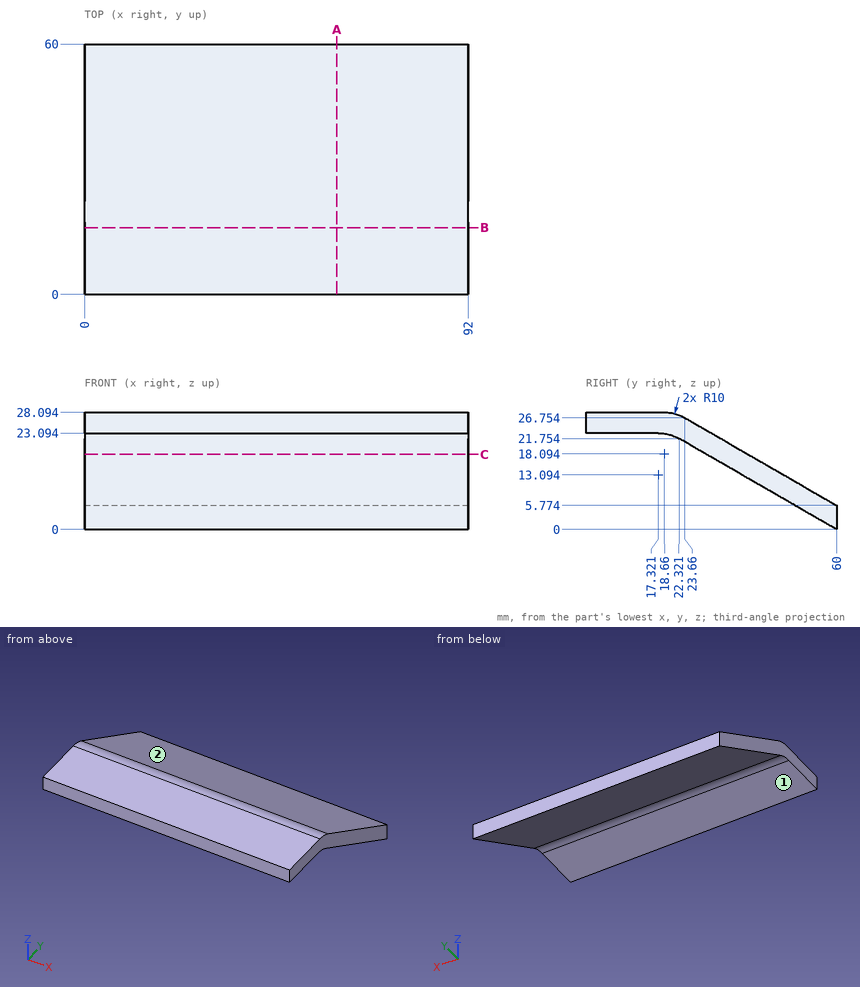
Part print with two shaded views. Sizes in mm from the minimum x, y, z corner. A direction names the side the tool comes from. Give positions to 0.01 mm unless a question says otherwise; leave off trailing zeros. Order: outer loops, then holes, each group sorted by start corner. A loop starts at its lowest first (then second) coordinate and runs counter-clockwise, first axis right, second up.
1) Pin check, flat tips, straight feed: pin 1 (6 mm diameter, centred on x = 39.5, y = 9.5, fed in from -Z); pin 2 (1.5 mm diameter, centred on x = 15, z = 14, fed in from +Y); pin 3 (4 mm diameter, centred on x = 48.5, z = 18, fed in from +Y) (1 decimal). Stop position of each tip, or through.
2) Saw through at A-A, the plane x = 60.5. Write the cut outline in (y, z) (1 decimal).
3) Wall check: probe 1 along Z at (x, y) = (60, 16.5) (1 decimal); probe 2 along Y at (x, z) = (33, 18.25); probe 3 along Z at (x, y) = (69.5, 22.5). Give the ranges that are in metal, low to high.
4) 3-axis set-ups, long thin cutter, end or side, ignore diameter. For the marked faces 1 and 2: which of +Z, -Z, +X, -X, +Y, -Y reach the whole face in a straight line?
5) Saw through at B-B, the plane y = 16. Write the cut outline in (x, z) (1 decimal).
6) Saw through at C-C, the plane z = 18. Write the cut outline in (x, y).
Computed:
1. pin 1: stops at z = 23.09
1. pin 2: stops at y = 47.05
1. pin 3: stops at y = 42.3
2. outline: (0, 23.1) - (17.3, 23.1) arc R10 cw to (22.3, 21.8) - (60, 0) - (60, 5.8) - (23.7, 26.8) arc R10 ccw to (18.7, 28.1) - (0, 28.1) - close
3. probe 1: z = 23.1 to 28.1
3. probe 2: y = 28.39 to 38.39
3. probe 3: z = 21.65 to 27.33
4. face 1: -Z, +X, -X, -Y
4. face 2: +Z, +X, -X, +Y
5. outline: (0, 23.1) - (92, 23.1) - (92, 28.1) - (0, 28.1) - close
6. outline: (0, 28.82) - (92, 28.82) - (92, 38.82) - (0, 38.82) - close
